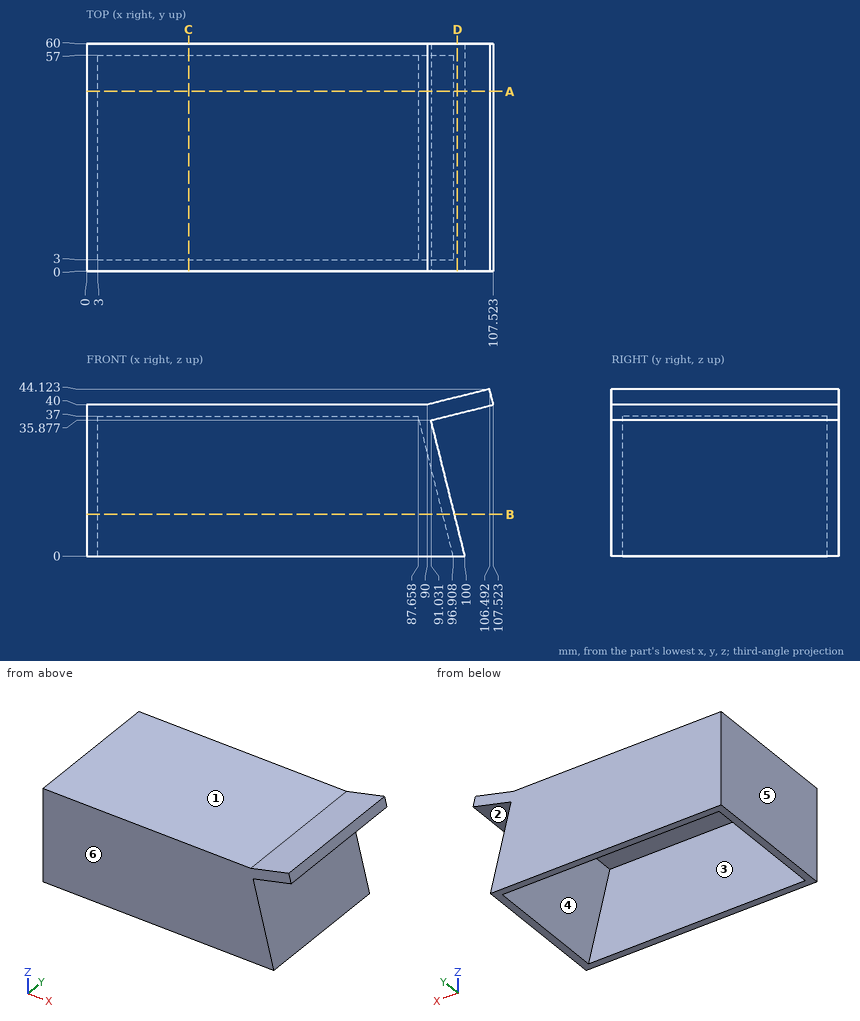
Here's the drawing with two shaded views (mm, measured from the low corner). I have some questions. A direction names the side the tool comes from. Coordinates: 2 decimals unless noted, no trailing zeros. Order: outer loops, then holes, each group sorted by start corner. A loop starts at its lowest first (then second) coordinate and runs counter-clockwise, first axis right, second up. Notation, with made-up numbers: (71.25, 80) - (124.25, 80) arc R18 ccw to (124.25, 114) - close; hole circle Ø4 at (-23.75, 42.5). An arc over 180 degrees is marked (long way). Use CSV: the item, a comma, the result in double quotes. Start each with the question number.
1. I'm going to push flat-ended pins straight in: pin 1 (3 mm diameter, centred on y = 43, z = 22, fed in from +X) (1 decimal); pin 2 (8 mm diameter, centred on x = 61, y = 32, fed in from -Z); pin 3 (18 mm diameter, centred on x = 24.5, y = 19.5, fed in from +Z). Where does each tip first touch, or does it pass through?
2. Suppose I cut it at D-D on x = 98. List the corners of the cut face in (y, z) for me.
3. Suppose I cut it at B-B on z = 11. List the corners of the cut face in (x, y) for me.
4. For the marked faces 1, 2 and 3, which set-ups out of +Z, -Z, +X, -X, +Y, -Y let a thin tool reach every point of the face, with its end or its side?
5. Please list where these lines run through material, in increasing order: line 1 (Y direction, x = 30.5, z = 27); line 2 (Z direction, x = 52, y = 11.5); line 3 (X direction, y = 49, z = 29). Write a range as from..to.
6. Suppose I cut it at A-A on y = 47.5. List the corners of the cut face in (x, z) for me.
7. If we mould it in two halves opening along Y, with no side actions, what happens to the marked faces 4, 5 and 6? For each: +Y half, -Y half, draft (parallel to the pull), parting line (faces both ways), or undercut.
8. Suppose I cut it at C-C on x = 27. List the corners of the cut face in (y, z) for me.
Output:
1,pin 1,"stops at x = 94.9"
1,pin 2,"stops at z = 37"
1,pin 3,"stops at z = 40"
2,outline,"(0, 0) - (60, 0) - (60, 8) - (0, 8) - close; (0, 37.62) - (60, 37.62) - (60, 42) - (0, 42) - close"
3,outline,"(0, 0) - (97.25, 0) - (97.25, 60) - (0, 60) - close; hole (3, 3) - (94.16, 3) - (94.16, 57) - (3, 57) - close"
4,face 1,"+Z, -X, +Y, -Y"
4,face 2,"+X, +Y, -Y"
4,face 3,"-Z"
5,line 1,"y = 0..3, 57..60"
5,line 2,"z = 37..40"
5,line 3,"x = 0..3, 89.66..92.75"
6,outline,"(0, 0) - (3, 0) - (3, 37) - (87.66, 37) - (96.91, 0) - (100, 0) - (91.03, 35.88) - (107.52, 40) - (106.49, 44.12) - (90, 40) - (0, 40) - close"
7,face 4,"undercut"
7,face 5,"draft"
7,face 6,"-Y half"
8,outline,"(0, 0) - (3, 0) - (3, 37) - (57, 37) - (57, 0) - (60, 0) - (60, 40) - (0, 40) - close"
